from build123d import *

# Parameters (mm, degrees)
F0_R     = 15.9511244513
F1_DEPTH = 21.336
F4_DEPTH = 4.572
F5_W     = 23.5527278855
F5_H     = 5.7727247477
F6_DEPTH = 19.304
F8_DEPTH = 62.23
F2_R     = 10.3729315348
F9_DEPTH = 46.99


with BuildPart() as f1:
    # F0 (on Top) → F1 (new body)
    with BuildSketch(Plane.XY):
        with Locations((31.4036346972, 31.5190926194)):
            Circle(F0_R)
    extrude(amount=F1_DEPTH)

    # F3 (on face) → F4 (join)
    with BuildSketch(Plane(origin=(0, 0, 0), x_dir=(1, 0, 0), z_dir=(0, 0, -1))):
        with BuildLine():
            Line((-9.6981814131, -47.4702170707), (31.4036346972, -47.4702170707))
            ThreePointArc((31.4036346972, -47.4702170707), (15.4525102459, -31.5190926194), (31.4036346972, -15.5679681681))
            Line((31.4036346972, -15.5679681681), (31.4036346972, -15.3554547578))
            Line((31.4036346972, -15.3554547578), (-9.6981814131, -15.3554547578))
            Line((-9.6981814131, -15.3554547578), (-9.6981814131, -47.4702170707))
        make_face()
    extrude(amount=-F4_DEPTH)

    # F5 (on face) → F6 (join)
    with BuildSketch(Plane(origin=(0, 0, 0), x_dir=(1, 0, 0), z_dir=(0, 0, -1))):
        with Locations((9.2363632284, -31.8654552102)):
            Rectangle(F5_W, F5_H)
    extrude(amount=-F6_DEPTH)

    # F7 (on face) → F8 (cut)
    with BuildSketch(Plane.XZ.offset(-28.9790928364)):
        Polygon((-2.5400007144, 19.304), (-2.5400007144, 4.572), (15.6560389326, 19.304), align=None)
    extrude(amount=-F8_DEPTH, mode=Mode.SUBTRACT)

    # F2 (on face) → F9 (cut)
    with BuildSketch(Plane.XY.offset(21.336)):
        with Locations((31.4036346972, 31.5190926194)):
            Circle(F2_R)
    extrude(amount=-F9_DEPTH, mode=Mode.SUBTRACT)


solid = f1.part
Here's how the part is built. I have some questions about the finished solid (model axes, mm). A direction names the side the tool comes from. Give positions to 0.01 mm unless a question says otherwise; leave off trailing zeros. Loops run counter-clockwise (first coordinate to the right, second up) from the corner with the lowest first, then second, coordinate; pieces in that order, holes last. Notation, with made-up numbers: (-25, 41.5) -> (-9, 41.5) arc R27 cw to (-9, 70.5) -> close; hole circle Ø8 at (81.25, -32.75). An arc over 180 degrees is marked (long way). One line per item, written item: value.
Q1. We'd pull the mould along X, two halves only. Please class faces 6 (the face through (40.986, 27.546, 10.817)), 7 (the face through (12, 31, 0)), 8 (the face through (46.14, 25.41, 10.52)): pulls with the +X half, pulls with the -X half, needs draft (parallel to the pull), parting line crosses it, or undercut.
Answers follow:
face 6: undercut
face 7: needs draft
face 8: parting line crosses it
Q2. Suppose I cut it at D-D on x = 5. Please give me the cut outline in (y, z).
Answers follow:
outline: (15.36, 0) -> (47.47, 0) -> (47.47, 4.57) -> (34.75, 4.57) -> (34.75, 10.68) -> (28.98, 10.68) -> (28.98, 4.57) -> (15.36, 4.57) -> close
Q3. Suppose I cut it at A-A on y = 40. Please give me the cut outline in (x, z), then the cut area to 3 significant figures.
Answers follow:
outline: (-9.7, 0) -> (25.43, 0) -> (25.43, 21.34) -> (17.89, 21.34) -> (17.89, 4.57) -> (-9.7, 4.57) -> close; (37.38, 0) -> (44.91, 0) -> (44.91, 21.34) -> (37.38, 21.34) -> close
area: 448 mm^2
Q4. On a 3-axis mill with a long thin cutter (end or side, diameter ignored), from which of +Z, -Z, +X, -X, +Y, -Y can I reach the whole of each face in a straight line? I mean faces 1 (the face through (6, 28, 4.572)), 2 (the face through (11, 15.355, 2)), 3 (the face through (10, 28.979, 9)), 4 (the face through (9, 34.752, 10)), 5 (the face through (-9.698, 31, 2)). Say none if no direction works.
Answers follow:
face 1: +Z, -X
face 2: +Z, -Z, +X, -X, -Y
face 3: +Z, -X, -Y
face 4: +Z, -X, +Y
face 5: +Z, -Z, -X, +Y, -Y
Q5. If I drill on line 1 along Y through (x, z) = (31, 15.25); line 2 along Y through (x, z) = (39.5, 13.5); line 3 along Z through (x, y) = (6.5, 21), over which ranges is the centre line in solid material (lowest first)?
Answers follow:
line 1: 15.57 to 21.15, 41.88 to 47.47
line 2: 17.78 to 25.03, 38 to 45.26
line 3: 0 to 4.57
Q6. Suppose I cut it at C-C on z = 3.25. Please give me the cut outline in (x, y), then the cut area to 3 significant figures.
Answers follow:
outline: (-9.7, 15.36) -> (31.4, 15.36) -> (31.4, 15.57) arc R15.95 ccw to (31.4, 47.47) -> (-9.7, 47.47) -> close; hole circle Ø20.75 at (31.4, 31.52)
area: 1,380 mm^2
Q7. I'm going to push flat-ended pins straight in: pin 1 Ø6 at (x, z) = (-2, 11) entering from +Y; pin 2 Ø8 at (x, y) = (40.5, 32.5) entering from +Z; pin 3 Ø5 at (x, z) = (30.5, 16) entering from -Y; pin 4 Ø8 at (x, y) = (-3, 28.5) entering from +Z. Where does each tip first touch, or does it pass through?
Answers follow:
pin 1: through
pin 2: z = 21.34
pin 3: y = 15.57
pin 4: z = 7.41
Q8. Suppose I cut it at B-B on x = 30. Please give me the cut outline in (y, z), then the cut area to 3 significant figures.
Answers follow:
outline: (15.36, 0) -> (21.24, 0) -> (21.24, 21.34) -> (15.63, 21.34) -> (15.63, 4.57) -> (15.36, 4.57) -> close; (41.8, 0) -> (47.47, 0) -> (47.47, 4.57) -> (47.41, 4.57) -> (47.41, 21.34) -> (41.8, 21.34) -> close
area: 241 mm^2
